Here's how the part is built. I have some questions about the finished solid (model axes, mm). A direction names the side the tool comes from. Round coordinates to 2 decimals unless told otherwise and drop trailing zeros. Write each loop counter-clockwise with the first axis right and the second up, starting at its lowest first coordinate (ties: lowest second). Pieces come first, ordered by that corner, then holes. Notation, with made-up numbers: (24.25, -7.75) -> (47.25, -7.75) arc R26 cw to (47.25, 23.25) -> close; hole circle Ø11 at (46, 39). An arc over 180 degrees is marked (long way). Answer in a Markdown table with one row per item.
from build123d import *

# Parameters (mm, degrees)
SKETCH1_W                             = 127
SKETCH1_H                             = 331.7875
BOSS_EXTRUDE1_DEPTH                   = 12.7
SKETCH9_R                             = 9.525
SKETCH9_R_2                           = 4.7625
CUT_EXTRUDE1_DEPTH                    = 339.048051549
CUT_EXTRUDE3_DEPTH                    = 3.175
F_10_CLEARANCE_HOLE2_D                = 5.1054
TAPPED_HOLE_FOR_10_32_HELICOIL1_D     = 5.1054
TAPPED_HOLE_FOR_10_32_HELICOIL1_DEPTH = 31.75
TAPPED_HOLE_FOR_10_32_HELICOIL1_TIP   = 1.533816902
F_1_4_CLEARANCE_HOLE1_D               = 6.7564


with BuildPart() as part:
    # Sketch1 → Boss-Extrude1 (new body)
    with BuildSketch(Plane(origin=(0, 0, 0), x_dir=(0, 0, -1), z_dir=(1, 0, 0))):
        with Locations((0, 165.89375)):
            Rectangle(SKETCH1_W, SKETCH1_H)
    extrude(amount=BOSS_EXTRUDE1_DEPTH)

    # Sketch9 → Cut-Extrude1 (cut, through all)
    with BuildSketch(Plane(origin=(12.7, 0, 0), x_dir=(0, 0, -1), z_dir=(1, 0, 0))):
        with Locations((39.6875, 309.5625)):
            Circle(SKETCH9_R)
        with Locations((39.6875, 227.0125)):
            Circle(SKETCH9_R)
        with Locations((33.3375, 268.2875)):
            Circle(SKETCH9_R_2)
    extrude(amount=-CUT_EXTRUDE1_DEPTH, mode=Mode.SUBTRACT)

    # Sketch24 → Cut-Extrude3 (cut)
    with BuildSketch(Plane.ZY):
        with BuildLine():
            Line((-42.8625, 296.8625), (-23.8125, 296.8625))
            ThreePointArc((-23.8125, 296.8625), (-19.322371939, 295.002628061), (-17.4625, 290.5125))
            Line((-17.4625, 290.5125), (-17.4625, 246.0625))
            ThreePointArc((-17.4625, 246.0625), (-19.322371939, 241.572371939), (-23.8125, 239.7125))
            Line((-23.8125, 239.7125), (-42.8625, 239.7125))
            ThreePointArc((-42.8625, 239.7125), (-47.352628061, 241.572371939), (-49.2125, 246.0625))
            Line((-49.2125, 246.0625), (-49.2125, 290.5125))
            ThreePointArc((-49.2125, 290.5125), (-47.352628061, 295.002628061), (-42.8625, 296.8625))
        make_face()
    extrude(amount=-CUT_EXTRUDE3_DEPTH, mode=Mode.SUBTRACT)

    # #10 Clearance Hole2 (through all)
    with Locations(Plane.ZY.offset(-3.175)):
        with Locations((-33.3375, 291.2999), (-33.3375, 245.2751)):
            Hole(F_10_CLEARANCE_HOLE2_D / 2)

    # Tapped Hole for #10-32 Helicoil1
    with Locations(Plane(origin=(0, 0, -63.5), x_dir=(-1, 0, 0), z_dir=(0, 0, -1))):
        with Locations((-6.35, 325.4375), (-6.35, 211.1375), (-6.35, 309.5625), (-6.35, 227.0125)):
            Hole(TAPPED_HOLE_FOR_10_32_HELICOIL1_D / 2, depth=TAPPED_HOLE_FOR_10_32_HELICOIL1_DEPTH)
            with Locations((0, 0, -(TAPPED_HOLE_FOR_10_32_HELICOIL1_DEPTH + TAPPED_HOLE_FOR_10_32_HELICOIL1_TIP / 2))):  # 118° drill point
                Cone(0, TAPPED_HOLE_FOR_10_32_HELICOIL1_D / 2, TAPPED_HOLE_FOR_10_32_HELICOIL1_TIP, mode=Mode.SUBTRACT)

    # 1/4 Clearance Hole1 (through all)
    with Locations(Plane(origin=(12.7, 0, 0), x_dir=(0, 0, -1), z_dir=(1, 0, 0))):
        with Locations((-52.3875, 25.4), (-26.9875, 50.8), (-52.3875, 50.8), (-26.9875, 25.4), (26.9875, 50.8), (52.3875, 25.4), (26.9875, 25.4), (52.3875, 50.8)):
            Hole(F_1_4_CLEARANCE_HOLE1_D / 2)


solid = part.part
1) I need wall thicknesses on line 1 (Y direction, x = 1.25, z = 53); line 2 (Y direction, x = 1.5, z = -42); line 3 (Y direction, x = 11, z = -43). Which ranges of each line are inside material? Lowest first, please. Write a range as [from, to].
Response:
| item | result |
|---|---|
| line 1 | y = [0, 22.08], [28.72, 47.48], [54.12, 331.79] |
| line 2 | y = [0, 217.77], [236.25, 239.71], [296.86, 300.32], [318.8, 331.79] |
| line 3 | y = [0, 218.08], [235.94, 300.63], [318.49, 331.79] |
2) I want a section at C-C, the plane y = 279.5. List the corners of the cut face in (x, z) for me (1 decimal).
Response:
| item | result |
|---|---|
| outline | (0, -63.5) -> (12.7, -63.5) -> (12.7, 63.5) -> (0, 63.5) -> (0, -17.5) -> (3.2, -17.5) -> (3.2, -49.2) -> (0, -49.2) -> close |
3) For pin 1 (6 mm diameter, centred on y = 245.28, z = -33.34, fed in from -X) (3 decimals), with a flat end and sliding along its axis, tell me the tip position at first contact or that it passes through.
Response:
| item | result |
|---|---|
| pin 1 | stops at x = 3.175 |
4) Which directions (+Z, -Z, +X, -X, +Y, -Y) give clear straight access to the entire face, cutting with the end or side of a thin tool? Please do faces 4 (the face through (1.57, 241.52, -47.3)), 5 (the face through (6.26, 54.15, 26.55)).
Response:
| item | result |
|---|---|
| face 4 | -X |
| face 5 | +X, -X |
5) We'd pull the mould along X, two halves only. Please class faces 1 (the face through (12.7, 168, 1)), 2 (the face through (3.175, 275, -33)), 3 (the face through (6.261, 23.344, -55.068)): +X half, -X half, draft (parallel to the pull), parting line (faces both ways), or undercut.
Response:
| item | result |
|---|---|
| face 1 | +X half |
| face 2 | -X half |
| face 3 | draft |
6) I want a section at B-B, the plane z = -52.5. List the corners of the cut face in (x, y) for me, and give its area (3 significant figures).
Response:
| item | result |
|---|---|
| outline | (0, 0) -> (12.7, 0) -> (12.7, 22.02) -> (0, 22.02) -> close; (0, 28.78) -> (12.7, 28.78) -> (12.7, 47.42) -> (0, 47.42) -> close; (0, 54.18) -> (12.7, 54.18) -> (12.7, 331.79) -> (0, 331.79) -> close; hole circle Ø5.11 at (6.35, 211.14); hole circle Ø5.11 at (6.35, 227.01); hole circle Ø5.11 at (6.35, 309.56); hole circle Ø5.11 at (6.35, 325.44) |
| area | 3,960 mm^2 |
7) I want a section at A-A, the plane y = 50.8. List the corners of the cut face in (x, z) for me.
Response:
| item | result |
|---|---|
| outline | (0, -63.5) -> (12.7, -63.5) -> (12.7, -55.77) -> (0, -55.77) -> close; (0, -49.01) -> (12.7, -49.01) -> (12.7, -30.37) -> (0, -30.37) -> close; (0, -23.61) -> (12.7, -23.61) -> (12.7, 23.61) -> (0, 23.61) -> close; (0, 30.37) -> (12.7, 30.37) -> (12.7, 49.01) -> (0, 49.01) -> close; (0, 55.77) -> (12.7, 55.77) -> (12.7, 63.5) -> (0, 63.5) -> close |
